```python
from build123d import *

# Parameters (mm, degrees)
ESQUISSE1_W             = 15
ESQUISSE1_H             = 20
BOSS_EXTRU_1_DEPTH      = 5
ESQUISSE2_W             = 5
ESQUISSE2_H             = 5
ESQUISSE2_R             = 2.25
ENL_V_MAT_EXTRU_1_DEPTH = 5
CONG_1_R                = 7.5
CONG_4_R                = 7.5
CONG_5_R                = 7


with BuildPart() as part:
    # Esquisse1 → Boss.-Extru.1 (new body)
    with BuildSketch(Plane.XY):
        with Locations((-45.477663375, -34.327294686)):
            Rectangle(ESQUISSE1_W, ESQUISSE1_H)
    extrude(amount=BOSS_EXTRU_1_DEPTH)

    # Esquisse2 → Enlèv. mat.-Extru.1 (cut)
    with BuildSketch(Plane.XY.offset(5)):
        with Locations((-45.477663375, -36.827294686)):
            Rectangle(ESQUISSE2_W, ESQUISSE2_H)
        with Locations((-45.477663375, -30.327294686)):
            Circle(ESQUISSE2_R)
    extrude(amount=-ENL_V_MAT_EXTRU_1_DEPTH, mode=Mode.SUBTRACT)

    # Congé1
    cong_1_edges = [part.edges().sort_by_distance(p)[0] for p in [
        (-52.977663375, -24.327294686, 2.5),
    ]]
    fillet(cong_1_edges, radius=CONG_1_R)

    # Congé4
    cong_4_edges = [part.edges().sort_by_distance(p)[0] for p in [
        (-37.977663375, -24.327294686, 2.5),
    ]]
    fillet(cong_4_edges, radius=CONG_4_R - 0.0001)  # a hair under: the kernel refuses the full size

    # Congé5
    cong_5_edges = [part.edges().sort_by_distance(p)[0] for p in [
        (-37.977663375, -44.327294686, 2.5),
        (-52.977663375, -44.327294686, 2.5),
    ]]
    fillet(cong_5_edges, radius=CONG_5_R)


solid = part.part
```
Here's how the part is built. I have some questions about the finished solid (model axes, mm). A direction names the side the tool comes from. Coordinates: 2 decimals unless noted, no trailing zeros. Write each loop counter-clockwise with the first axis right and the second up, starting at its lowest first coordinate (ties: lowest second). Pieces come first, ordered by that corner, then holes. Notation, with made-up numbers: (5.25, 46.25) - (19.25, 46.25) arc R28 ccw to (19.25, 79.25) - close; hole circle Ø10 at (85.25, -17). An arc over 180 degrees is marked (long way). One line per item, written item: value.
1) Suppose I cut it at D-D on y = -40.5. Write out the boundary of the cut face in (x, z), and give its area (3 significant figures).
Model answer:
outline: (-52.22, 0) - (-38.74, 0) - (-38.74, 5) - (-52.22, 5) - close
area: 67.4 mm²
2) Suppose I cut it at A-A on y = -36. Write out the boundary of the cut face in (x, z).
Model answer:
outline: (-52.98, 0) - (-47.98, 0) - (-47.98, 5) - (-52.98, 5) - close; (-42.98, 0) - (-37.98, 0) - (-37.98, 5) - (-42.98, 5) - close
3) On a 3-axis mill with a long thin cutter (end or side, diameter ignored), from which of +Z, -Z, +X, -X, +Y, -Y can I reach the whole of each face in a straight line? I mean faces 1 (the flat face through (-47.978, -37, 3)), 2 (the flat face through (-37.978, -35, 2)). Say none if no direction works.
Model answer:
face 1: +Z, -Z
face 2: +Z, -Z, +X, +Y, -Y
4) Suppose I cut it at C-C on x = -43.75. Write out the boundary of the cut face in (y, z), and give its area (3 significant figures).
Model answer:
outline: (-44.22, 0) - (-39.33, 0) - (-39.33, 5) - (-44.22, 5) - close; (-34.33, 0) - (-31.77, 0) - (-31.77, 5) - (-34.33, 5) - close; (-28.89, 0) - (-24.53, 0) - (-24.53, 5) - (-28.89, 5) - close
area: 59.0 mm²
5) Suppose I cut it at B-B on z = 4.2. State how many separate pieces and enclosed holes the cut face has, and give its area (3 significant figures).
Model answer:
separate pieces: 1
enclosed holes: 2
area: 214 mm²
6) We'd pull the mould along X, two halves only. Please class faces 3 (the cylindrical face through (-39.97, -42.22, 2.54)), 4 (the flat face through (-52.978, -35, 2)), 5 (the flat face through (-45.5, -44.327, 2.5)), 6 (the flat face through (-46, -39.327, 3)): pulls with the +X half, pulls with the -X half, needs draft (parallel to the pull), parting line crosses it, or undercut.
Model answer:
face 3: pulls with the +X half
face 4: pulls with the -X half
face 5: needs draft
face 6: undercut
7) I'm going to push a flat-ended pin straight in: P1, Ø2, axis at y = -27.5, z = 2.5, coming from the +X side. Where does the tip first touch, or does it pass through?
Model answer:
P1: stops at x = -38.76
8) I need wall thicknesses on line 1 along Y through (x, z) = (-47.25, 0.95); line 2 along X through (y, z) = (-34.75, 0.85); line 3 along Y through (x, z) = (-45.25, 2.9). Which ranges of each line are inside material? Lowest first, please.
Model answer:
line 1: y = -44.21 to -39.33, -34.33 to -31.71, -28.94 to -24.54
line 2: x = -52.98 to -47.98, -42.98 to -37.98
line 3: y = -44.33 to -39.33, -34.33 to -32.57, -28.09 to -24.33
